Geometry check sheet. Reference: drawing and pictorial views, mm from the part's lowest x, y, z. A direction names the side the tool comes from. Round coordinates to 2 decimals unless told otherwise and drop trailing zeros. Loops run counter-clockwise (first coordinate to the right, second up) from the corner with the lowest first, then second, coordinate; pieces in that order, holes last. Notation, with made-up numbers: (49.25, 17) -> (63.25, 17) arc R12 ccw to (63.25, 37) -> close; hole circle Ø10 at (64, 14). An arc over 180 degrees is marked (long way). Use one line per item in the form item = value.
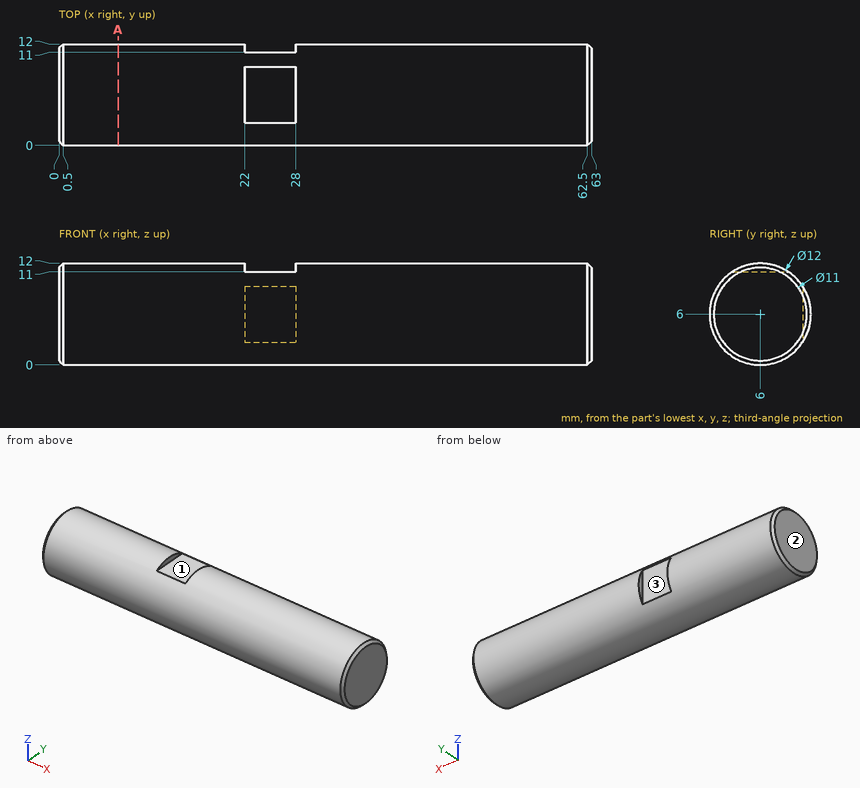
1. Gauge pin test, flat ends, axial feed: pin 1 (1.5 mm diameter, centred on x = 17.5, z = 1.5, fed in from -Y); pin 2 (1 mm diameter, centred on x = 43, z = 5, fed in from -Y); pin 3 (1.8 mm diameter, centred on x = 26.5, z = 7.5, fed in from +Y). Record the tip position at first contact, or that the pin passes through.
Return value:
pin_1 = 1.32
pin_2 = 0.02
pin_3 = 11
2. Material ranges on line 1 along Y through (x, z) = (20, 1); line 2 along Y through (x, z) = (34.5, 6.5); line 3 along Z through (x, y) = (49.5, 8.75), recorded low to high.
Return value:
line_1 = 2.68 to 9.32
line_2 = 0.02 to 11.98
line_3 = 0.67 to 11.33
3. Section check A-A (x = 7). Record the boundary of the cut face in (y, z).
Return value:
outline = circle Ø12 at (6, 6)
4. Tool access check on the marked faces 1, 2 and 3. Record the directions out of +Z, -Z, +X, -X, +Y, -Y that give a thin tool (end or side, any length) a straight path to the whole face; none if there is none.
Return value:
face_1 = +Z, +Y, -Y
face_2 = +Z, -Z, -X, +Y, -Y
face_3 = +Z, -Z, +Y
